Build history of the part. All positions in model axes, mm. Give positions to 0.01 mm unless a question says otherwise; leave off trailing zeros. Order: outer loops, then holes, each group sorted by start corner. A loop starts at its lowest first (then second) coordinate and runs counter-clockwise, first axis right, second up. Notation, with made-up numbers: (27.25, -9.75) - (54.25, -9.75) arc R10 cw to (54.25, 3.25) - close; hole circle Ø11 at (43.25, 21). An arc over 180 degrees is marked (long way). One line per item, written item: value.
```python
from build123d import *

# Parameters (mm, degrees)
RESSALTO_EXTRUS_O1_DEPTH = 5
FURO_COM_FOLGA_DE_M61_D  = 6.6
FURO_COM_FOLGA_DE_M51_D  = 5.5
RESSALTO_EXTRUS_O3_DEPTH = 5
CORTE_EXTRUS_O1_DEPTH    = 419.231218825
ESBO_O19_W               = 20
ESBO_O19_H               = 18
CORTE_EXTRUS_O2_DEPTH    = 385.449518663


with BuildPart() as part:
    # Esboço1 → Ressalto-extrusão1 (new body)
    with BuildSketch(Plane.XY):
        Polygon((0, 76.5), (0, 132.32), (0, 172.82), (116, 172.82), (116, 134.82), (244, 134.82), (244, 172.82), (360, 172.82), (360, 132.32), (360, 76.5), (350, 76.5), (350, 46.5), (360, 46.5), (360, 0), (195, 0), (195, 8), (165, 8), (165, 0), (0, 0), (0, 46.5), (10, 46.5), (10, 76.5), align=None)
    extrude(amount=RESSALTO_EXTRUS_O1_DEPTH)

    # Furo com folga de M61 (through all)
    with Locations(Plane(origin=(-158.278165294, -245.41916969, 5), x_dir=(-1, 0, 0), z_dir=(0, 0, 1))):
        with Locations((-163.278165294, -331.91916969), (-163.278165294, -270.06916969), (-513.278165294, -331.91916969), (-513.278165294, -270.06916969), (-458.278165294, -374.23916969), (-428.278165294, -374.23916969), (-248.278165294, -374.23916969), (-218.278165294, -374.23916969), (-335.278165294, -374.23916969), (-163.278165294, -346.91916969), (-513.278165294, -346.91916969), (-310.278165294, -374.23916969)):
            Hole(FURO_COM_FOLGA_DE_M61_D / 2)

    # Furo com folga de M51 (through all)
    with Locations(Plane(origin=(-158.278165294, -245.41916969, 5), x_dir=(-1, 0, 0), z_dir=(0, 0, 1))):
        with Locations((-470.278165294, -297.91916969), (-470.278165294, -262.41916969), (-206.278165294, -297.91916969), (-206.278165294, -262.41916969), (-465.278165294, -249.41916969), (-440.278165294, -249.41916969), (-358.278165294, -249.41916969), (-318.278165294, -249.41916969), (-236.278165294, -249.41916969), (-211.278165294, -249.41916969)):
            Hole(FURO_COM_FOLGA_DE_M51_D / 2)

    # Esboço15 → Ressalto-extrusão3 (add, through all)
    with BuildSketch(Plane.XY.offset(5)):
        Polygon((100, 172.82), (100, 212.82), (0, 172.82), align=None)
        Polygon((260, 172.82), (260, 212.82), (360, 172.82), align=None)
    extrude(amount=-RESSALTO_EXTRUS_O3_DEPTH)

    # Esboço18 → Corte-extrusão1 (cut, through all)
    with BuildSketch(Plane.XY.offset(5)):
        Polygon((118, 134.82), (118, 123), (0, 123), (0, 223), (360, 223), (360, 123), (242, 123), (242, 134.82), align=None)
    extrude(amount=-CORTE_EXTRUS_O1_DEPTH, mode=Mode.SUBTRACT)

    # Esboço19 → Corte-extrusão2 (cut, through all)
    with BuildSketch(Plane.XY.offset(5)):
        with Locations((217, 125.82)):
            Rectangle(ESBO_O19_W, ESBO_O19_H)
    extrude(amount=-CORTE_EXTRUS_O2_DEPTH, mode=Mode.SUBTRACT)


solid = part.part
```
(1) Drill centre lines: line 1 (Y direction, x = 48, z = 1.95); line 2 (Y direction, x = 355, z = 3.4); line 3 (X direction, y = 128.82, z = 1.3). Where is each one in solid material? Low to high.
Completed:
line 1: 0 to 14.25, 19.75 to 49.75, 55.25 to 123
line 2: 0 to 21.35, 27.95 to 46.5, 76.5 to 83.2, 89.8 to 98.2, 104.8 to 123
line 3: 118 to 148.7, 155.3 to 173.7, 180.3 to 207, 227 to 242
(2) Slice it at B-B, the plane x = 177. Give the cut face in (y, z), and give its area (3 significant figures).
Completed:
outline: (8, 0) - (125.52, 0) - (125.52, 5) - (8, 5) - close; (132.12, 0) - (134.82, 0) - (134.82, 5) - (132.12, 5) - close
area: 601 mm²
(3) Slice it at D-D, the plane x = 109. Give the cut face in (y, z), and give its area (3 significant figures).
Completed:
outline: (0, 0) - (123, 0) - (123, 5) - (0, 5) - close
area: 615 mm²
(4) Pull direction Y, two halves, no side cores. Call faces 1 (the face through (4.57, 83.23, 2.46)), 2 (the face through (177, 68, 0)): +Y half, -Y half, draft (parallel to the pull), parting line (faces both ways), or undercut.
Completed:
face 1: undercut
face 2: draft
(5) Slice it at C-C, the plane z = 2.95. Count the separate pieces of the cut face and the enclosed holes in it, and give its area (3 significant figures).
Completed:
separate pieces: 1
enclosed holes: 18
area: 44,000 mm²
(6) Slice it at A-A, the plane x = 5. Give the cut face in (y, z).
Completed:
outline: (0, 0) - (21.35, 0) - (21.35, 5) - (0, 5) - close; (27.95, 0) - (46.5, 0) - (46.5, 5) - (27.95, 5) - close; (76.5, 0) - (83.2, 0) - (83.2, 5) - (76.5, 5) - close; (89.8, 0) - (98.2, 0) - (98.2, 5) - (89.8, 5) - close; (104.8, 0) - (123, 0) - (123, 5) - (104.8, 5) - close
(7) Pin check, flat tips, straight feed: P1, Ø1.5, axis at y = 59.5, z = 2.5, coming from the -X side; P2, Ø9, axis at x = 200, y = 4, coming from the +Z side; P3, Ø2.5, axis at y = 67, z = 2.5, coming from the +X side; P4, Ø1.5, axis at y = 129, z = 3.5, coming from the +X side. Stop position of each tip, or through.
Completed:
P1: x = 10
P2: z = 5
P3: x = 350
P4: x = 242
